```python
from build123d import *

# Parameters (mm, degrees)
F0_R     = 3.175
F1_DEPTH = 3.175


# Not quite as in the source:
# - a length typed as a fraction of an inch, garbled in the dataset ("3 / 203.2 mm" for 3/8 in), is restored


with BuildPart() as f1:
    # F0 (on Top) → F1 (new body)
    with BuildSketch(Plane.XY):
        with BuildLine():
            ThreePointArc((-63.5, -7.62), (-62.0121024484, -11.2121024484), (-58.42, -12.7))
            Line((-58.42, -12.7), (-38.1, -12.7))
            ThreePointArc((-38.1, -12.7), (-20.1394877579, -20.1394877579), (-12.7, -38.1))
            Line((-12.7, -38.1), (-12.7, -58.42))
            ThreePointArc((-12.7, -58.42), (-11.2121024484, -62.0121024484), (-7.62, -63.5))
            Line((-7.62, -63.5), (0, -63.5))
            Line((0, -63.5), (7.62, -63.5))
            ThreePointArc((7.62, -63.5), (11.2121024484, -62.0121024484), (12.7, -58.42))
            Line((12.7, -58.42), (12.7, -38.1))
            ThreePointArc((12.7, -38.1), (20.1394877579, -20.1394877579), (38.1, -12.7))
            Line((38.1, -12.7), (58.42, -12.7))
            ThreePointArc((58.42, -12.7), (62.0121024484, -11.2121024484), (63.5, -7.62))
            Line((63.5, -7.62), (63.5, 0))
            Line((63.5, 0), (63.5, 7.62))
            ThreePointArc((63.5, 7.62), (62.0121024484, 11.2121024484), (58.42, 12.7))
            Line((58.42, 12.7), (38.1, 12.7))
            ThreePointArc((38.1, 12.7), (20.1394877579, 20.1394877579), (12.7, 38.1))
            Line((12.7, 38.1), (12.7, 58.42))
            ThreePointArc((12.7, 58.42), (11.2121024484, 62.0121024484), (7.62, 63.5))
            Line((7.62, 63.5), (-7.62, 63.5))
            ThreePointArc((-7.62, 63.5), (-11.2121024484, 62.0121024484), (-12.7, 58.42))
            Line((-12.7, 58.42), (-12.7, 38.1))
            ThreePointArc((-12.7, 38.1), (-20.1394877579, 20.1394877579), (-38.1, 12.7))
            Line((-38.1, 12.7), (-58.42, 12.7))
            ThreePointArc((-58.42, 12.7), (-62.0121024484, 11.2121024484), (-63.5, 7.62))
            Line((-63.5, 7.62), (-63.5, 0))
            Line((-63.5, 0), (-63.5, -7.62))
        make_face()
        with Locations((0, -50.8)):
            Circle(F0_R, mode=Mode.SUBTRACT)
        with Locations((0, -25.4)):
            Circle(F0_R, mode=Mode.SUBTRACT)
        with Locations((-50.8, 0)):
            Circle(F0_R, mode=Mode.SUBTRACT)
        with Locations((-25.4, 0)):
            Circle(F0_R, mode=Mode.SUBTRACT)
        with Locations((25.4, 0)):
            Circle(F0_R, mode=Mode.SUBTRACT)
        with Locations((0, 25.4)):
            Circle(F0_R, mode=Mode.SUBTRACT)
        with Locations((50.8, 0)):
            Circle(F0_R, mode=Mode.SUBTRACT)
        with Locations((0, 50.8)):
            Circle(F0_R, mode=Mode.SUBTRACT)
    extrude(amount=F1_DEPTH)


solid = f1.part
```
Read the model definition and answer for the solid it produces. Units are mm, in the model's axes. A direction names the side the tool comes from. Round coordinates to 2 decimals unless told otherwise and drop trailing zeros. Write each loop counter-clockwise with the first axis right and the second up, starting at its lowest first coordinate (ties: lowest second). Pieces come first, ordered by that corner, then holes. Notation, with made-up numbers: (59.5, 31) - (81.5, 31) arc R27 ccw to (81.5, 53) - close; hole circle Ø1 at (27.5, 64.25). An arc over 180 degrees is marked (long way). Use CSV: the item, a comma, the result in double quotes.
Q1. Each of these flat-tipped pins is pushed along its axis until it touches: pin 1 Ø4 at (x, y) = (-25.4, 0) entering from -Z; pin 2 Ø1 at (x, z) = (-50, 2) entering from +Y; pin 3 Ø1.6 at (y, z) = (49.5, 1.5) entering from +X; pin 4 Ø1.6 at (y, z) = (-47.5, 1.5) entering from -X. Where does it stop, or does it pass through?
Values:
pin 1,"passes through"
pin 2,"stops at y = 12.7"
pin 3,"stops at x = 12.7"
pin 4,"stops at x = -12.7"
Q2. Find section B-B, the plane y = -25.4. Write down the section's boundary in (x, z) (3 decimals), then the cut area to 3 significant figures.
Values:
outline,"(-16.103, 0) - (-3.175, 0) - (-3.175, 3.175) - (-16.103, 3.175) - close; (3.175, 0) - (16.103, 0) - (16.103, 3.175) - (3.175, 3.175) - close"
area,"82.1 mm²"
Q3. Find section D-D, the plane x = -49.5. Write down the section's boundary in (y, z) (3 decimals), then the cut area to 3 significant figures.
Values:
outline,"(-12.7, 0) - (-2.897, 0) - (-2.897, 3.175) - (-12.7, 3.175) - close; (2.897, 0) - (12.7, 0) - (12.7, 3.175) - (2.897, 3.175) - close"
area,"62.3 mm²"
Q4. Find section A-A, the plane x = 0. Write down the section's boundary in (y, z) (3 decimals), then the cut area to 3 significant figures.
Values:
outline,"(-63.5, 0) - (-53.975, 0) - (-53.975, 3.175) - (-63.5, 3.175) - close; (-47.625, 0) - (-28.575, 0) - (-28.575, 3.175) - (-47.625, 3.175) - close; (-22.225, 0) - (22.225, 0) - (22.225, 3.175) - (-22.225, 3.175) - close; (28.575, 0) - (47.625, 0) - (47.625, 3.175) - (28.575, 3.175) - close; (53.975, 0) - (63.5, 0) - (63.5, 3.175) - (53.975, 3.175) - close"
area,"323 mm²"
Q5. A tool of negligible diameter and unlimited length cuts with its end or side. For faces 5 (the flat face through (-48, -12.7, 2)), 6 (the flat face through (-48, 12.7, 2)), 7 (the flat face through (12.7, -48, 2)), from which of +Z, -Z, +X, -X, +Y, -Y can it reach the whole face along a straight path? Write none if from no direction.
Values:
face 5,"+Z, -Z, -X, -Y"
face 6,"+Z, -Z, -X, +Y"
face 7,"+Z, -Z, +X, -Y"
Q6. Straight lines are drawn through the part: line 1 along Y through (x, z) = (0, 1.5) (3 decimals); line 2 along Y through (x, z) = (-44, 1.7). For each, find the intervals that lie inside material, in ascending order.
Values:
line 1,"y = -63.5 to -53.975, -47.625 to -28.575, -22.225 to 22.225, 28.575 to 47.625, 53.975 to 63.5"
line 2,"y = -12.7 to 12.7"
Q7. Find section C-C, the plane z = 1.55. Count the separate pieces of the cut face and the enclosed holes in it, then the cut area to 3 significant figures.
Values:
separate pieces,"1"
enclosed holes,"8"
area,"6,060 mm²"
Q8. Determine the mould class of faces 1 (the cylindrical face through (1.707, -48.123, 1.565)), 2 (the cylindrical face through (-0.41, -22.25, 1.57)), 3 (the cylindrical face through (-61.972, 11.251, 1.565)), 4 (the flat face through (48, -12.7, 2)) for opening direction X: +X half, -X half, draft (parallel to the pull), parting line (faces both ways), or undercut.
Values:
face 1,"undercut"
face 2,"undercut"
face 3,"-X half"
face 4,"draft"
